Design review of the part built by this model. Coordinates are the model's own, in mm. Face numbers are marked on the shaded views. A direction names the side the tool comes from. Coordinates: 2 decimals unless noted, no trailing zeros. Order: outer loops, then holes, each group sorted by start corner. A loop starts at its lowest first (then second) coordinate and runs counter-clockwise, first axis right, second up. Notation, with made-up numbers: (42, 10.5) -> (59, 10.5) arc R13 cw to (59, 16.5) -> close; hole circle Ø4 at (-13.75, -30). An arc over 180 degrees is marked (long way). Write item = value, one per line.
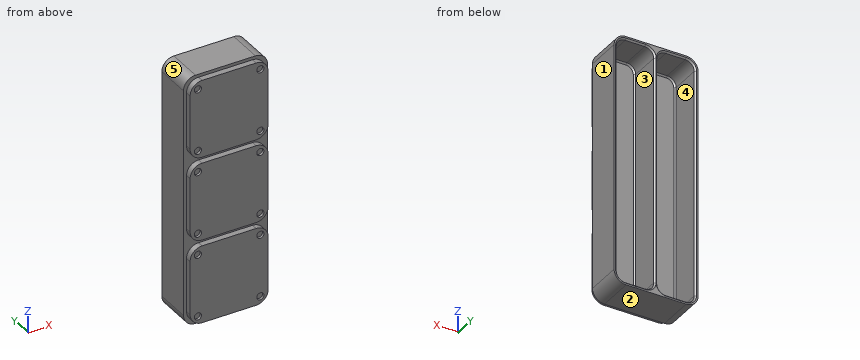
```python
from build123d import *

# Parameters (mm, degrees)
BOSS_EXTRUDE4_DEPTH = 5
SKETCH7_R           = 3
CUT_EXTRUDE4_DEPTH  = 2
SKETCH8_W           = 70
SKETCH8_H           = 70
BOSS_EXTRUDE5_DEPTH = 30
MIRROR2_START       = 5
MIRROR2_OUTLINE_W   = 70
MIRROR2_OUTLINE_H   = 70
MIRROR2_DEPTH       = 30
MIRROR2_2_OUTLINE_R = 3
MIRROR2_2_DEPTH     = 5
MIRROR2_START_2     = 2
MIRROR2_3_OUTLINE_R = 3
MIRROR2_3_DEPTH     = 3
FILLET1_R           = 10
CUT_EXTRUDE5_DEPTH  = 30
BOSS_EXTRUDE6_DEPTH = 2.5
BOSS_EXTRUDE7_DEPTH = 27.5
FILLET2_R           = 7.5
CHAMFER1_SIZE       = 1.25


# Read off the part's stored shape, not the designer's step: Mirror2
with BuildPart() as part:
    # Sketch5 → Boss-Extrude4 (new body)
    with BuildSketch(Plane(origin=(0, 0, 0), x_dir=(1, 0, 0), z_dir=(0, 1, 0))):
        with BuildLine():
            Line((-22.5, -32.5), (22.5, -32.5))
            ThreePointArc((22.5, -32.5), (29.571067812, -29.571067812), (32.5, -22.5))
            Line((32.5, -22.5), (32.5, 22.5))
            ThreePointArc((32.5, 22.5), (29.571067812, 29.571067812), (22.5, 32.5))
            Line((22.5, 32.5), (-22.5, 32.5))
            ThreePointArc((-22.5, 32.5), (-29.571067812, 29.571067812), (-32.5, 22.5))
            Line((-32.5, 22.5), (-32.5, -22.5))
            ThreePointArc((-32.5, -22.5), (-29.571067812, -29.571067812), (-22.5, -32.5))
        make_face()
    extrude(amount=BOSS_EXTRUDE4_DEPTH)

    # Sketch7 → Cut-Extrude4 (cut)
    with BuildSketch(Plane.XZ):
        with Locations(Location((-26.035533906, 26.035533906, 0), (0, 0, 270))):
            Circle(SKETCH7_R)
        with Locations(Location((26.036533906, 26.036533906, 0), (0, 0, 270))):
            Circle(SKETCH7_R)
        with Locations(Location((26.037533906, -26.035533906, 0), (0, 0, 270))):
            Circle(SKETCH7_R)
        with Locations(Location((-26.034533906, -26.036533906, 0), (0, 0, 270))):
            Circle(SKETCH7_R)
    extrude(amount=-CUT_EXTRUDE4_DEPTH, mode=Mode.SUBTRACT)

    # Sketch8 → Boss-Extrude5 (add)
    with BuildSketch(Plane(origin=(0, 5, 0), x_dir=(1, 0, 0), z_dir=(0, 1, 0))):
        Rectangle(SKETCH8_W, SKETCH8_H)
    extrude(amount=BOSS_EXTRUDE5_DEPTH)

    # Mirror2 outline → Mirror2 (add)
    with BuildSketch(Plane(origin=(0, 0, 0), x_dir=(1, 0, 0), z_dir=(0, 1, 0)).offset(MIRROR2_START)):
        with Locations((0, -70)):
            Rectangle(MIRROR2_OUTLINE_W, MIRROR2_OUTLINE_H)
        with Locations((0, 70)):
            Rectangle(MIRROR2_OUTLINE_W, MIRROR2_OUTLINE_H)
    extrude(amount=MIRROR2_DEPTH)

    # Mirror2 2 outline → Mirror2 2 (add)
    # profile 1 of 2: a face of its own
    with BuildSketch(Plane(origin=(0, 0, 0), x_dir=(1, 0, 0), z_dir=(0, 1, 0))):
        with BuildLine():
            Line((32.5, -92.5), (32.5, -47.5))
            ThreePointArc((32.5, -47.5), (29.571067812, -40.428932188), (22.5, -37.5))
            Line((22.5, -37.5), (-22.5, -37.5))
            ThreePointArc((-22.5, -37.5), (-29.571067812, -40.428932188), (-32.5, -47.5))
            Line((-32.5, -47.5), (-32.5, -92.5))
            ThreePointArc((-32.5, -92.5), (-29.571067812, -99.571067812), (-22.5, -102.5))
            Line((-22.5, -102.5), (22.5, -102.5))
            ThreePointArc((22.5, -102.5), (29.571067812, -99.571067812), (32.5, -92.5))
        make_face()
        with Locations((-26.034533906, -96.036533906)):
            Circle(MIRROR2_2_OUTLINE_R, mode=Mode.SUBTRACT)
        with Locations((-26.035533906, -43.964466094)):
            Circle(MIRROR2_2_OUTLINE_R, mode=Mode.SUBTRACT)
        with Locations((26.037533906, -96.035533906)):
            Circle(MIRROR2_2_OUTLINE_R, mode=Mode.SUBTRACT)
        with Locations((26.036533906, -43.963466094)):
            Circle(MIRROR2_2_OUTLINE_R, mode=Mode.SUBTRACT)
    # profile 2 of 2: a face of its own
    with BuildSketch(Plane(origin=(0, 0, 0), x_dir=(1, 0, 0), z_dir=(0, 1, 0))):
        with BuildLine():
            Line((32.5, 47.5), (32.5, 92.5))
            ThreePointArc((32.5, 92.5), (29.571067812, 99.571067812), (22.5, 102.5))
            Line((22.5, 102.5), (-22.5, 102.5))
            ThreePointArc((-22.5, 102.5), (-29.571067812, 99.571067812), (-32.5, 92.5))
            Line((-32.5, 92.5), (-32.5, 47.5))
            ThreePointArc((-32.5, 47.5), (-29.571067812, 40.428932188), (-22.5, 37.5))
            Line((-22.5, 37.5), (22.5, 37.5))
            ThreePointArc((22.5, 37.5), (29.571067812, 40.428932188), (32.5, 47.5))
        make_face()
        with Locations((-26.034533906, 43.963466094)):
            Circle(MIRROR2_2_OUTLINE_R, mode=Mode.SUBTRACT)
        with Locations((-26.035533906, 96.035533906)):
            Circle(MIRROR2_2_OUTLINE_R, mode=Mode.SUBTRACT)
        with Locations((26.037533906, 43.964466094)):
            Circle(MIRROR2_2_OUTLINE_R, mode=Mode.SUBTRACT)
        with Locations((26.036533906, 96.036533906)):
            Circle(MIRROR2_2_OUTLINE_R, mode=Mode.SUBTRACT)
    extrude(amount=MIRROR2_2_DEPTH)

    # Mirror2 3 outline → Mirror2 3 (add)
    with BuildSketch(Plane(origin=(0, 0, 0), x_dir=(1, 0, 0), z_dir=(0, 1, 0)).offset(MIRROR2_START_2)):
        with Locations((-26.035533906, -43.964466094)):
            Circle(MIRROR2_3_OUTLINE_R)
        with Locations((26.036533906, -43.963466094)):
            Circle(MIRROR2_3_OUTLINE_R)
        with Locations((26.037533906, -96.035533906)):
            Circle(MIRROR2_3_OUTLINE_R)
        with Locations((-26.034533906, -96.036533906)):
            Circle(MIRROR2_3_OUTLINE_R)
        with Locations((-26.035533906, 96.035533906)):
            Circle(MIRROR2_3_OUTLINE_R)
        with Locations((26.036533906, 96.036533906)):
            Circle(MIRROR2_3_OUTLINE_R)
        with Locations((26.037533906, 43.964466094)):
            Circle(MIRROR2_3_OUTLINE_R)
        with Locations((-26.034533906, 43.963466094)):
            Circle(MIRROR2_3_OUTLINE_R)
    extrude(amount=MIRROR2_3_DEPTH)

    # Fillet1
    fillet1_edges = [part.edges().sort_by_distance(p)[0] for p in [
        (35, 20, 105),
        (-35, 20, 105),
        (-35, 20, -105),
        (35, 20, -105),
    ]]
    fillet(fillet1_edges, radius=FILLET1_R)

    # Sketch9 → Cut-Extrude5 (cut)
    with BuildSketch(Plane(origin=(0, 35, 0), x_dir=(1, 0, 0), z_dir=(0, 1, 0))):
        with BuildLine():
            Line((-32.5, 95), (-32.5, -95))
            ThreePointArc((-32.5, -95), (-30.303300859, -100.303300859), (-25, -102.5))
            Line((-25, -102.5), (25, -102.5))
            ThreePointArc((25, -102.5), (30.303300859, -100.303300859), (32.5, -95))
            Line((32.5, -95), (32.5, 95))
            ThreePointArc((32.5, 95), (30.303300859, 100.303300859), (25, 102.5))
            Line((25, 102.5), (-25, 102.5))
            ThreePointArc((-25, 102.5), (-30.303300859, 100.303300859), (-32.5, 95))
        make_face()
    extrude(amount=-CUT_EXTRUDE5_DEPTH, mode=Mode.SUBTRACT)


with BuildPart() as cut_extrude5_piece_1:
    # of the separate pieces the step leaves, piece 1, a body of its own (cut_extrude5_pieces)
    add(part.part.solids().sort_by_distance((35, 5, 95))[0])



with BuildPart() as cut_extrude5_piece_2:
    # of the separate pieces the step leaves, piece 2, a body of its own (cut_extrude5_pieces)
    add(part.part.solids().sort_by_distance((32.5, 0, 92.5))[0])


with BuildPart() as cut_extrude5_piece_3:
    # of the separate pieces the step leaves, piece 3, a body of its own (cut_extrude5_pieces)
    add(part.part.solids().sort_by_distance((32.5, 0, -47.5))[0])


with BuildPart() as cut_extrude5_piece_4:
    # of the separate pieces the step leaves, piece 4, a body of its own (cut_extrude5_pieces)
    add(part.part.solids().sort_by_distance((32.5, 0, 22.5))[0])


with BuildPart() as cut_extrude5_piece_1_1:
    add(cut_extrude5_piece_1.part)

    add(cut_extrude5_piece_2.part)  # Boss-Extrude6 merges Cut-Extrude5 piece 2

    add(cut_extrude5_piece_3.part)  # Boss-Extrude6 merges Cut-Extrude5 piece 3

    add(cut_extrude5_piece_4.part)  # Boss-Extrude6 merges Cut-Extrude5 piece 4
    # Sketch10 → Boss-Extrude6 (add)
    with BuildSketch(Plane.XZ.offset(-5)):
        with BuildLine():
            Line((25, 105), (-25, 105))
            ThreePointArc((-25, 105), (-32.071067812, 102.071067812), (-35, 95))
            Line((-35, 95), (-35, -95))
            ThreePointArc((-35, -95), (-32.071067812, -102.071067812), (-25, -105))
            Line((-25, -105), (25, -105))
            ThreePointArc((25, -105), (32.071067812, -102.071067812), (35, -95))
            Line((35, -95), (35, 95))
            ThreePointArc((35, 95), (32.071067812, 102.071067812), (25, 105))
        make_face()
    extrude(amount=-BOSS_EXTRUDE6_DEPTH)

    # Sketch11 → Boss-Extrude7 (add)
    with BuildSketch(Plane(origin=(0, 35, 0), x_dir=(1, 0, 0), z_dir=(0, 1, 0))):
        Polygon((-1.25, -102.5), (1.25, -102.5), (1.25, 102.5), (0, 102.5), (-1.25, 102.5), align=None)
    extrude(amount=-BOSS_EXTRUDE7_DEPTH)

    # Fillet2
    fillet2_edges = [cut_extrude5_piece_1_1.edges().sort_by_distance(p)[0] for p in [
        (-1.25, 21.25, 102.5),
        (1.25, 21.25, 102.5),
        (1.25, 21.25, -102.5),
        (-1.25, 21.25, -102.5),
    ]]
    fillet(fillet2_edges, radius=FILLET2_R)

    # Chamfer1
    chamfer1_edges = [cut_extrude5_piece_1_1.edges().sort_by_distance(p)[0] for p in [
        (-16.875, 35, 102.5),
        (-32.5, 35, 0),
        (-30.303300859, 35, 100.303300859),
        (30.303300859, 35, 100.303300859),
        (30.303300859, 35, -100.303300859),
        (-30.303300859, 35, -100.303300859),
        (1.25, 7.5, 0),
        (1.25, 35, 0),
        (16.875, 7.5, 102.5),
        (3.446699141, 7.5, 100.303300859),
        (3.446699141, 7.5, -100.303300859),
        (16.875, 35, 102.5),
        (-1.25, 7.5, 0),
        (-1.25, 35, 0),
        (-16.875, 7.5, -102.5),
        (-3.446699141, 7.5, -100.303300859),
        (-3.446699141, 7.5, 100.303300859),
        (-16.875, 35, -102.5),
        (3.446699141, 35, -100.303300859),
        (3.446699141, 35, 100.303300859),
        (-3.446699141, 35, 100.303300859),
        (-3.446699141, 35, -100.303300859),
        (-30.303300859, 7.5, -100.303300859),
        (-16.875, 7.5, 102.5),
        (30.303300859, 7.5, 100.303300859),
        (32.5, 7.5, 0),
        (30.303300859, 7.5, -100.303300859),
        (16.875, 7.5, -102.5),
        (-32.5, 7.5, 0),
        (-30.303300859, 7.5, 100.303300859),
        (16.875, 35, -102.5),
        (32.5, 35, 0),
    ]]
    chamfer(chamfer1_edges, length=CHAMFER1_SIZE - 0.0001)  # a hair under: the kernel refuses the full size


solid = cut_extrude5_piece_1_1.part
```
(1) For the marked faces 4 and 5, list the 3-axis set-ups (+Z, -Z, +X, -X, +Y, -Y) from which the entire face can be reached by the end or side of a thin tool; tool diameter is ignored.
Report:
face_4 = +Y
face_5 = +Z, -X, +Y, -Y
(2) For L1, parallel to X at y = 10.5, z = 46.5; L2, parallel to Z at x = -16, y = 2; L3, parallel to Z at x = -13.5, y = 21, list the stretches that pass through material, from the lowest coordinate up.
Report:
L1 = -35 to -32.5, -1.25 to 1.25, 32.5 to 35
L2 = -102.5 to -37.5, -32.5 to 32.5, 37.5 to 102.5
L3 = -105 to -102.5, 102.5 to 105
(3) We need section C-C (x = -17). Write out the cut boundary in (y, z), and give its area (3 significant figures).
Report:
outline = (0, -102.5) -> (5, -102.5) -> (5, -105) -> (35, -105) -> (35, -103.75) -> (33.75, -102.5) -> (8.75, -102.5) -> (7.5, -101.25) -> (7.5, 101.25) -> (8.75, 102.5) -> (33.75, 102.5) -> (35, 103.75) -> (35, 105) -> (5, 105) -> (5, 102.5) -> (0, 102.5) -> (0, 37.5) -> (5, 37.5) -> (5, 32.5) -> (0, 32.5) -> (0, -32.5) -> (5, -32.5) -> (5, -37.5) -> (0, -37.5) -> close
area = 1,640 mm²
(4) The part is to be moulded in two halves that separate along X. For the marked faces 1, 2 and 3, say which applies: released by +X, released by -X, zero draft, split by the parting line, or undercut.
Report:
face_1 = released by +X
face_2 = zero draft
face_3 = undercut
(5) We need section B-B (y = 13). Write out the cut boundary in (x, z).
Report:
outline = (-35, -95) arc R10 ccw to (-25, -105) -> (25, -105) arc R10 ccw to (35, -95) -> (35, 95) arc R10 ccw to (25, 105) -> (-25, 105) arc R10 ccw to (-35, 95) -> close; hole (-32.5, -95) arc R7.5 ccw to (-25, -102.5) -> (-8.75, -102.5) arc R7.5 ccw to (-1.25, -95) -> (-1.25, 95) arc R7.5 ccw to (-8.75, 102.5) -> (-25, 102.5) arc R7.5 ccw to (-32.5, 95) -> close; hole (1.25, -95) arc R7.5 ccw to (8.75, -102.5) -> (25, -102.5) arc R7.5 ccw to (32.5, -95) -> (32.5, 95) arc R7.5 ccw to (25, 102.5) -> (8.75, 102.5) arc R7.5 ccw to (1.25, 95) -> close
(6) Insertion check: pin 1 (2.5 mm diameter, centred on y = 3, z = -73, fed in from +X); pin 2 (10 mm diameter, centred on x = 7, z = 84, fed in from +Y); pin 3 (3.5 mm diameter, centred on x = -26.04, z = 43.96, fed in from -Y). Each pin has a flat end and moves straight along its axis. Give the tip position at first contact, or say it passes through.
Report:
pin_1 = 32.5
pin_2 = 8
pin_3 = 2
